The listing builds one solid part. Answer for the finished solid, in the listing's coordinates (mm). A direction names the side the tool comes from. Give positions to 0.01 mm unless a question says otherwise; leave off trailing zeros. Write each loop counter-clockwise with the first axis right and the second up, starting at its lowest first coordinate (ties: lowest second). Pieces come first, ordered by that corner, then holes. Notation, with made-up numbers: (-33.75, -5) -> (-18.75, -5) arc R23 cw to (-18.75, 4) -> close; hole circle Ø4 at (-4, 2.5). An arc over 180 degrees is marked (long way). Use CSV: the item, a comma, the result in double quotes. Start each with the question number.
from build123d import *

# Parameters (mm, degrees)
F0_W     = 609.6
F0_H     = 508
F0_W_2   = 266.7
F0_H_2   = 203.2
F1_DEPTH = 12.7
F2_W     = 609.6
F2_H     = 508
F2_W_2   = 294.601322
F2_H_2   = 224.288658
F3_DEPTH = 6.35


with BuildPart() as f1:
    # F0 (on Top) → F1 (new body)
    with BuildSketch(Plane.XY):
        Rectangle(F0_W, F0_H)
        with Locations((0, 133.655697)):
            Rectangle(F0_W_2, F0_H_2, mode=Mode.SUBTRACT)
    extrude(amount=F1_DEPTH)

    # F2 (on face) → F3 (join)
    with BuildSketch(Plane.XY.offset(12.7)):
        Rectangle(F2_W, F2_H)
        with Locations((0, 133.950159)):
            Rectangle(F2_W_2, F2_H_2, mode=Mode.SUBTRACT)
    extrude(amount=F3_DEPTH)


solid = f1.part
Q1. The mould has two halves that part along X. Classify faces 4 (the face through (304.8, -4, 9)), 5 (the face through (133.35, 132, 6)), 6 (the face through (-304.8, -4, 9)): +X half, -X half, draft (parallel to the pull), parting line (faces both ways), or undercut.
Q2. Straight lines are drawn through the part: L1, parallel to Y at x = 63.5, z = 6.5; L2, parallel to Y at x = 121.5, z = 14.75; L3, parallel to X at y = 196.5, z = 9.75. For each, find the intervals that lie inside material, in ascending order.
Q3. A flat-ended cylindrical pin translates along its axis: pin 1 Ø10 at (x, y) = (119, -187) entering from -Z. Find the tip coordinate at first contact, or state that the pin passes through.
Q4. Section A-A on x = -96 is taken. Give the vertices of the cut face in (y, z), then the cut area to 3 significant figures.
Q5. Section C-C on z = 3 is taken. Give the vertices of the cut face in (x, y).
Q6. For faces 1 (the face through (-12, 26, 12.7)), 2 (the face through (-2, 32.056, 6)), 3 (the face through (-4, -53, 19.05)), determine the directions among +Z, -Z, +X, -X, +Y, -Y from which every point of the face is accessible in a straight line to the end or side of a thin tool.
Q7. Section B-B on y = 205.5 is taken. Give the vertices of the cut face in (x, z).
Output:
1,face 4,"+X half"
1,face 5,"undercut"
1,face 6,"-X half"
2,L1,"-254 to 32.06, 235.26 to 254"
2,L2,"-254 to 21.81, 246.09 to 254"
2,L3,"-304.8 to -133.35, 133.35 to 304.8"
3,pin 1,"z = 0"
4,outline,"(-254, 0) -> (32.06, 0) -> (32.06, 12.7) -> (21.81, 12.7) -> (21.81, 19.05) -> (-254, 19.05) -> close; (235.26, 0) -> (254, 0) -> (254, 19.05) -> (246.09, 19.05) -> (246.09, 12.7) -> (235.26, 12.7) -> close"
4,area,"5,670 mm²"
5,outline,"(-304.8, -254) -> (304.8, -254) -> (304.8, 254) -> (-304.8, 254) -> close; hole (-133.35, 32.06) -> (133.35, 32.06) -> (133.35, 235.26) -> (-133.35, 235.26) -> close"
6,face 1,"+Z"
6,face 2,"+Z, -Z"
6,face 3,"+Z, +X, -X, +Y, -Y"
7,outline,"(-304.8, 0) -> (-133.35, 0) -> (-133.35, 12.7) -> (-147.3, 12.7) -> (-147.3, 19.05) -> (-304.8, 19.05) -> close; (133.35, 0) -> (304.8, 0) -> (304.8, 19.05) -> (147.3, 19.05) -> (147.3, 12.7) -> (133.35, 12.7) -> close"
